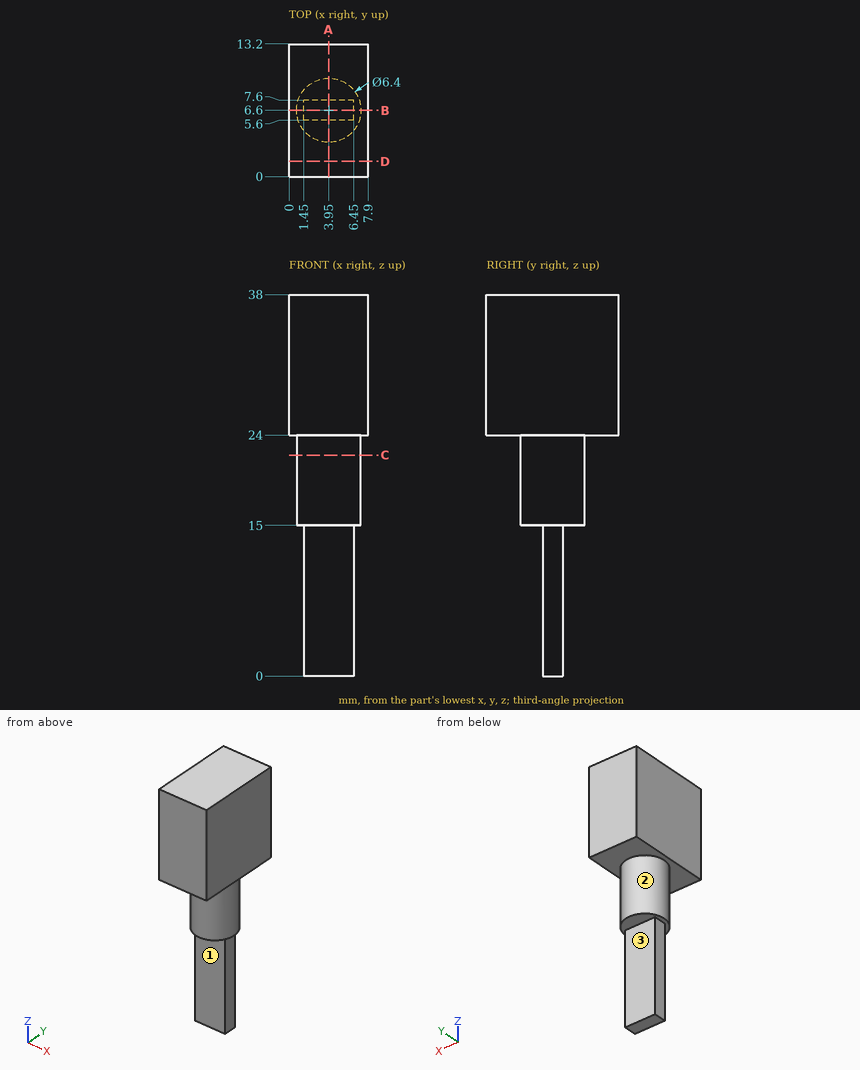
The figure shows three views and two pictorial views of one solid part (mm, origin at its lowest corner). Answer the questions. A direction names the side the tool comes from. Give positions to 0.01 mm unless a question says otherwise; leave off trailing zeros. Order: outer loops, then holes, each group sorted by start corner. A loop starts at its lowest first (then second) coordinate and runs counter-clockwise, first axis right, second up. Notation, with made-up numbers: M 34,88 L 67,88 A24 cw 67,105 Z; hole C -16.5,-16.5 d6. An arc over 180 degrees is marked long. Return JSON: item names as keys, results as strings.
Q1. Find the intervals of material crossed by line 1 along X through (y, z) = (7.25, 10.5); line 2 along Y through (x, z) = (3.75, 16); line 3 along Y through (x, z) = (6, 12), in increasing order. Write a range as [from, to].
Answer below:
{"line 1": "x = [1.45, 6.45]", "line 2": "y = [3.41, 9.79]", "line 3": "y = [5.6, 7.6]"}
Q2. Find section B-B, the plane y = 6.6. Write down the section's boundary in (x, z).
Answer below:
{"outline": "M 0,24 L 0.75,24 L 0.75,15 L 1.45,15 L 1.45,0 L 6.45,0 L 6.45,15 L 7.15,15 L 7.15,24 L 7.9,24 L 7.9,38 L 0,38 Z"}
Q3. Find section A-A, the plane x = 3.95. Write down the section's boundary in (y, z).
Answer below:
{"outline": "M 0,24 L 3.4,24 L 3.4,15 L 5.6,15 L 5.6,0 L 7.6,0 L 7.6,15 L 9.8,15 L 9.8,24 L 13.2,24 L 13.2,38 L 0,38 Z"}
Q4. Each of these flat-tipped pins is pushed along its axis until it touches: pin 1 (1.5 mm diameter, centred on x = 4.5, z = 8.5, fed in from +Y); pin 2 (1.5 mm diameter, centred on x = 1, z = 23, fed in from +Y); pin 3 (4 mm diameter, centred on x = 5, z = 4.5, fed in from -Y). Where does it stop, or does it pass through?
Answer below:
{"pin 1": "stops at y = 7.6", "pin 2": "stops at y = 8.92", "pin 3": "stops at y = 5.6"}
Q5. Find section C-C, the plane z = 22. Write down the section's boundary in (x, y).
Answer below:
{"outline": "C 3.95,6.6 d6.4"}
Q6. Find section D-D, the plane y = 1.5. Write down the section's boundary in (x, z).
Answer below:
{"outline": "M 0,24 L 7.9,24 L 7.9,38 L 0,38 Z"}
Q7. Which of the six approach directions +Z, -Z, +X, -X, +Y, -Y give full straight-line access (tool end or side, diameter ignored) to the marked faces 1, 2 and 3?
Answer below:
{"face 1": "-Z, +X, -X, -Y", "face 2": "-Z", "face 3": "-Z, +X, -X, +Y"}
